Check sheet for the modelled part. Datum: model origin and axes. Units: mm. A direction names the side the tool comes from. Round coordinates to 2 decimals unless told otherwise and drop trailing zeros. Loops run counter-clockwise (first coordinate to the right, second up) from the corner with the lowest first, then second, coordinate; pieces in that order, holes last. Notation, with made-up numbers: (37.25, 3) -> (84.25, 3) arc R25 cw to (84.25, 24) -> close; hole circle Ø10 at (-8, -1.5). An arc over 180 degrees is marked (long way). One line per item, written item: value. Start each with the question number.
1. Cross-section at B-B on x = 23.5. Record the cut outline in (y, z).
2. Go/stop test with a flat-tipped pin: pin 1 (2 mm diameter, centred on x = 32, y = 79, fed in from +Z). Record where the tip stops, or that it passes through.
3. Set-up check for faces 1 (the face through (51, 85, 16)), 2 (the face through (65.58, 4.69, 20.19)), 3 (the face through (23, 4, 9.931)), 4 (the face through (35, 89.027, 14)): record each of +Z, -Z, +X, -X, +Y, -Y from which the full face is reachable in a straight line by a thin tool's end or side.
4. Cross-section at C-C on z = 23.5. Record the cut outline in (x, y), then the cut area to 3 significant figures.
5. Release check for a two-part mould opening along X. For faces 5 (the face through (35, 81.407, 18)), 6 (the face through (34, 0, 14)), 7 (the face through (4, 85, 11.176)) record: +X half, -X half, draft (parallel to the pull), parting line (faces both ways), or undercut.
6. Cross-section at D-D on y = 32. Record the cut outline in (x, z).
7. Material ranges on L1, parallel to X at y = 3.81, z = 18.75; L2, parallel to X at y = 3.81, z = 22; L3, parallel to Y at x = 60, z = 27.25, recorded low to high.
8. Cross-section at A-A on y = 3.81. Record the cut outline in (x, z).
Autodesk Inventor part; units mm, degrees
ref_plane "YZ Plane" through (0, 0, 0) normal (1, 0, 0) x (0, 1, 0)
ref_plane "XZ Plane" through (0, 0, 0) normal (0, 1, 0) x (-1, 0, 0)
ref_plane "XY Plane" through (0, 0, 0) normal (0, 0, 1) x (1, 0, 0)
sketch "Sketch8" plane through (0, 0, 0) normal (0, 0, 1) x (1, 0, 0)
  line L0 (0, 0) -> (68.834, 0)
  line L1 (68.834, 0) -> (68.834, 89.027)
  line L2 (68.834, 89.027) -> (0, 89.027)
  line L3 (0, 89.027) -> (0, 0)
  dimension "d20" = 89.027
  dimension "d21" = 68.834
extrude "Extrusion6" add sketch "Sketch8" along normal blind 28.956
shell "Shell2" thickness 7.62 removed faces 1 at (45.8893, 29.6757, 28.956)
sketch "Sketch9" plane through (0, 0, 0) normal (0, -1, 0) x (1, 0, 0)
  point P0 (0, 0)
sketch "Sketch10" plane through (0, 0, 0) normal (0, -1, 0) x (1, 0, 0)
  line L0 (16.51, 20.5994) -> (29.21, 20.5994)
  line L1 (29.21, 20.5994) -> (29.21, 9.9314)
  line L2 (29.21, 9.9314) -> (16.51, 9.9314)
  line L3 (16.51, 9.9314) -> (16.51, 20.5994)
  line L4 (0, 0) -> (68.834, 0)
  line L5 (0, 0) -> (0, 28.956)
  line L6 (48.26, 20.9296) -> (57.15, 20.9296)
  line L7 (57.15, 20.9296) -> (57.15, 9.9314)
  line L8 (57.15, 9.9314) -> (48.26, 9.9314)
  line L9 (48.26, 9.9314) -> (48.26, 20.9296)
  line L10 (68.834, 0) -> (68.834, 28.956)
  dimension "d25" = 10.668
  dimension "d26" = 12.7
  dimension "d27" = 9.9314
  dimension "d28" = 16.51
  dimension "d29" = 10.9982
  dimension "d30" = 8.89
  dimension "d31" = 9.9314
  dimension "d32" = 11.684
extrude "Extrusion7" cut sketch "Sketch10" against normal blind 28.956 contours L0 L1 L2 L3
extrude "Extrusion8" cut sketch "Sketch10" against normal blind 28.956 contours L6 L7 L8 L9
sketch "Sketch11" plane through (7.62, 81.407, 7.62) normal (0, -1, 0) x (1, 0, 0)
  point P0 (-7.62, -7.62)
sketch "Sketch12" plane through (0, 89.027, 0) normal (0, 1, 0) x (1, 0, 0)
  circle A0 centre (48.514, -16.256) radius 2.5
  line L0 (68.834, 0) -> (68.834, -28.956)
  line L1 (68.834, -28.956) -> (0, -28.956)
  point P0 (0, 0)
  dimension "d37" = 5
  dimension "d38" = 20.32
  dimension "d39" = 12.7
extrude "Extrusion9" cut sketch "Sketch12" against normal blind 28.956
sketch "Sketch13" plane through (0, 0, 28.956) normal (0, 0, 1) x (1, 0, 0)
  line L0 (0, 89.027) -> (0, 0)
  line L1 (0, 89.027) -> (7.62, 81.407)
  circle A0 centre (3.81, 85.217) radius 1.0414
  line L2 (7.62, 81.407) -> (61.214, 81.407)
  line L3 (61.214, 81.407) -> (68.834, 89.027)
  line L4 (7.62, 7.62) -> (61.214, 7.62)
  line L5 (7.62, 7.62) -> (0, 0)
  line L6 (0, 0) -> (68.834, 0)
  line L7 (61.214, 7.62) -> (68.834, 0)
  circle A1 centre (65.024, 85.217) radius 1.0414
  circle A2 centre (3.81, 3.81) radius 1.0414
  circle A3 centre (65.024, 3.81) radius 1.0414
  dimension "d42" = 2.0828
  dimension "d43" = 2.0828
  dimension "d44" = 2.0828
  dimension "d45" = 2.0828
extrude "Extrusion10" cut sketch "Sketch13" against normal blind 17.78 contours A0 L1 | L1 A0
extrude "Extrusion11" cut sketch "Sketch13" against normal blind 17.78 contours A1 L3 | L3 A1
extrude "Extrusion12" cut sketch "Sketch13" against normal blind 17.78 contours A2 L5 | L5 A2
extrude "Extrusion13" cut sketch "Sketch13" against normal blind 17.78 contours A3 L7 | L7 A3
sketch "Sketch14" plane through (0, 89.027, 0) normal (0, 1, 0) x (1, 0, 0)
  line L0 (21.2173, -18.756) -> (10.5493, -18.756)
  line L1 (10.5493, -18.756) -> (10.5493, -13.168)
  line L2 (10.5493, -13.168) -> (21.2173, -13.168)
  line L3 (21.2173, -13.168) -> (21.2173, -18.756)
  circle A0 centre (48.514, -16.256) radius 2.5
  point P0 (0, 0)
  dimension "d54" = 10.668
  dimension "d55" = 5.588
  dimension "d56" = 0
extrude "Extrusion14" cut sketch "Sketch14" against normal blind 17.78 contours L0 L1 L2 L3
properties part number "arduinoCase"
Taken from the geometry:
1. outline: (0, 0) -> (89.03, 0) -> (89.03, 28.96) -> (81.41, 28.96) -> (81.41, 7.62) -> (7.62, 7.62) -> (7.62, 9.93) -> (0, 9.93) -> close; (0, 20.6) -> (7.62, 20.6) -> (7.62, 28.96) -> (0, 28.96) -> close
2. pin 1: stops at z = 7.62
3. face 1: +Y
3. face 2: +Z
3. face 3: -Y
3. face 4: +Z, -Z, +X, -X, +Y
4. outline: (0, 0) -> (68.83, 0) -> (68.83, 89.03) -> (0, 89.03) -> close; hole circle Ø2.08 at (3.81, 3.81); hole circle Ø2.08 at (3.81, 85.22); hole (7.62, 7.62) -> (61.21, 7.62) -> (61.21, 81.41) -> (7.62, 81.41) -> close; hole circle Ø2.08 at (65.02, 3.81); hole circle Ø2.08 at (65.02, 85.22)
4. area: 2,160 mm2
5. face 5: undercut
5. face 6: draft
5. face 7: undercut
6. outline: (0, 0) -> (68.83, 0) -> (68.83, 28.96) -> (61.21, 28.96) -> (61.21, 7.62) -> (7.62, 7.62) -> (7.62, 28.96) -> (0, 28.96) -> close
7. L1: x = 0 to 2.77, 4.85 to 16.51, 29.21 to 48.26, 57.15 to 63.98, 66.07 to 68.83
7. L2: x = 0 to 2.77, 4.85 to 63.98, 66.07 to 68.83
7. L3: y = 0 to 7.62, 81.41 to 89.03
8. outline: (0, 0) -> (68.83, 0) -> (68.83, 28.96) -> (66.07, 28.96) -> (66.07, 11.18) -> (63.98, 11.18) -> (63.98, 28.96) -> (4.85, 28.96) -> (4.85, 11.18) -> (2.77, 11.18) -> (2.77, 28.96) -> (0, 28.96) -> close; hole (16.51, 9.93) -> (29.21, 9.93) -> (29.21, 20.6) -> (16.51, 20.6) -> close; hole (48.26, 9.93) -> (57.15, 9.93) -> (57.15, 20.93) -> (48.26, 20.93) -> close
